Part print with two shaded views. Sizes in mm from the minimum x, y, z corner. Round coordinates to 2 decimals unless told otherwise and drop trailing zeros. Loops run counter-clockwise (first coordinate to the right, second up) from the corner with the lowest first, then second, coordinate; pieces in that order, holes last. Notation, with made-up numbers: M 39,15 L 83,15 A24 ccw 83,26 Z; hole C -40,85 d3. An arc over 180 degrees is marked long. Use a Markdown table: item, result. Add a question column.
Item 1: Saw through at C-C on z = 0.9. Write the cut outline in (x, y).
Item 2: Wall check: L1, parallel to X at y = 12.5, z = 2.5; L2, parallel to Y at x = 15, z = 2.4; L3, parallel to X at y = 14.5, z = 5.2. Give the ranges that are in metal, low to high. Write a range as from..to.
Item 3: Saw through at B-B on x = 115. Write the cut outline in (y, z), then the cut area to 3 significant figures.
Item 4: Saw through at A-A on y = 12.5. Write the cut outline in (x, z), then the cut area to 3 significant figures.
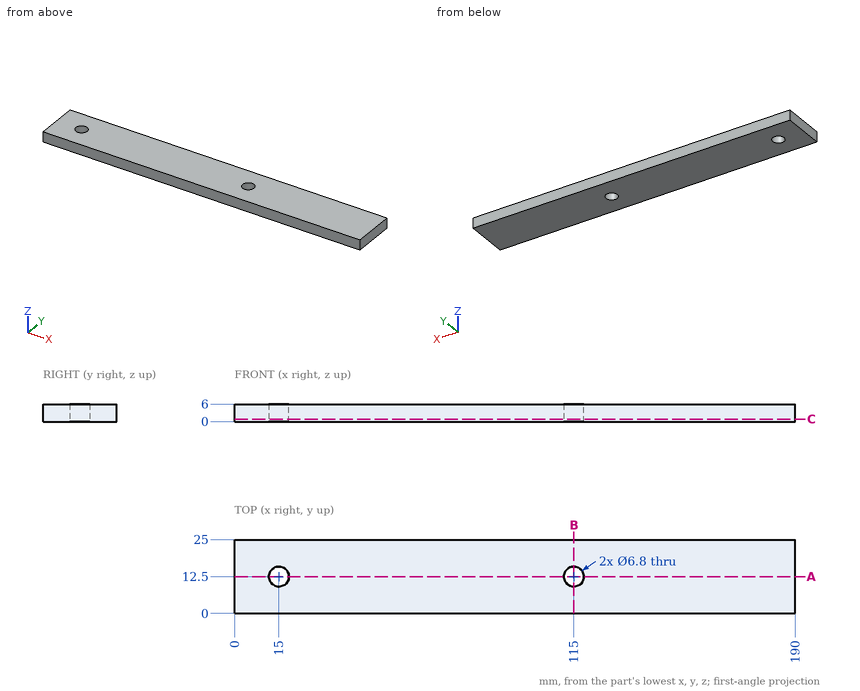
Entries:
| question | item | result |
|---|---|---|
| 1 | outline | M 0,0 L 190,0 L 190,25 L 0,25 Z; hole C 15,12.5 d6.8; hole C 115,12.5 d6.8 |
| 2 | L1 | 0..11.6, 18.4..111.6, 118.4..190 |
| 2 | L2 | 0..9.1, 15.9..25 |
| 2 | L3 | 0..12.25, 17.75..112.25, 117.75..190 |
| 3 | outline | M 0,0 L 9.1,0 L 9.1,6 L 0,6 Z; M 15.9,0 L 25,0 L 25,6 L 15.9,6 Z |
| 3 | area | 109 mm2 |
| 4 | outline | M 0,0 L 11.6,0 L 11.6,6 L 0,6 Z; M 18.4,0 L 111.6,0 L 111.6,6 L 18.4,6 Z; M 118.4,0 L 190,0 L 190,6 L 118.4,6 Z |
| 4 | area | 1,060 mm2 |
